Check sheet for the modelled part. Datum: model origin and axes. Units: mm. Face numbers are marked on the shaded views. A direction names the side the tool comes from. Round coordinates to 2 decimals unless told otherwise and drop trailing zeros. Order: outer loops, then holes, each group sorted by start corner. A loop starts at its lowest first (then second) coordinate and runs counter-clockwise, first axis right, second up.
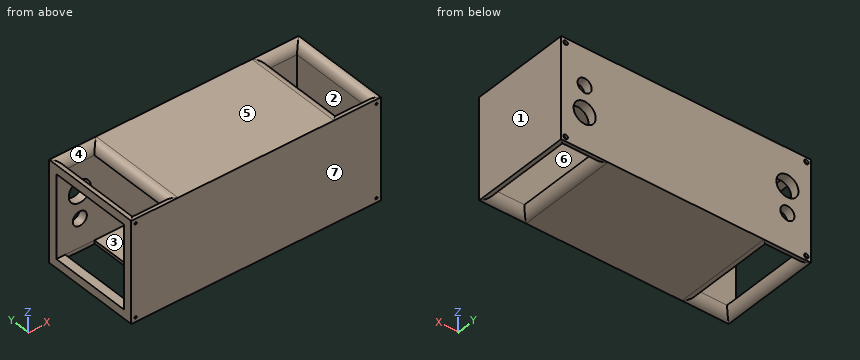
```python
from build123d import *

# Parameters (mm, degrees)
SKETCH1_W           = 282.5
SKETCH1_H           = 114
BOSS_EXTRUDE1_DEPTH = 114
SKETCH5_W           = 33
SKETCH5_H           = 94
CUT_EXTRUDE3_DEPTH  = 326.266429255
SKETCH6_W           = 94
SKETCH6_H           = 94
CUT_EXTRUDE4_DEPTH  = 262
SKETCH7_R           = 1.25
CUT_EXTRUDE5_DEPTH  = 262
SKETCH8_R           = 2.5
CUT_EXTRUDE6_DEPTH  = 2.5
FILLET3_R           = 10
FILLET4_R           = 10
FILLET6_R           = 10
SKETCH11_R          = 8
SKETCH11_R_2        = 12.5
CUT_EXTRUDE7_DEPTH  = 10


with BuildPart() as part:
    # Sketch1 → Boss-Extrude1 (new body)
    with BuildSketch(Plane.XY):
        with Locations((-141.25, 57)):
            Rectangle(SKETCH1_W, SKETCH1_H)
    extrude(amount=BOSS_EXTRUDE1_DEPTH)

    # Sketch5 → Cut-Extrude3 (cut, through all)
    with BuildSketch(Plane.XY):
        with Locations((-256, 57)):
            Rectangle(SKETCH5_W, SKETCH5_H)
        with Locations((-26.5, 57)):
            Rectangle(SKETCH5_W, SKETCH5_H)
    extrude(amount=CUT_EXTRUDE3_DEPTH, mode=Mode.SUBTRACT)

    # Sketch6 → Cut-Extrude4 (cut)
    with BuildSketch(Plane.ZY.offset(282.5)):
        with Locations((57, 57)):
            Rectangle(SKETCH6_W, SKETCH6_H)
    extrude(amount=-CUT_EXTRUDE4_DEPTH, mode=Mode.SUBTRACT)

    # Sketch7 → Cut-Extrude5 (cut)
    with BuildSketch(Plane(origin=(0, 114, 0), x_dir=(1, 0, 0), z_dir=(0, 1, 0))):
        with Locations(Location((-277.5, -109, 0), (0, 0, 180))):
            Circle(SKETCH7_R)
        with Locations(Location((-277.5, -5, 0), (0, 0, 180))):
            Circle(SKETCH7_R)
        with Locations(Location((-5, -109, 0), (0, 0, 180))):
            Circle(SKETCH7_R)
        with Locations(Location((-5, -5, 0), (0, 0, 180))):
            Circle(SKETCH7_R)
    extrude(amount=-CUT_EXTRUDE5_DEPTH, mode=Mode.SUBTRACT)

    # Sketch8 → Cut-Extrude6 (cut)
    with BuildSketch(Plane(origin=(0, 114, 0), x_dir=(1, 0, 0), z_dir=(0, 1, 0))):
        with Locations(Location((-277.5, -5, 0), (0, 0, 180))):
            Circle(SKETCH8_R)
        with Locations((-277.5, -109)):
            Circle(SKETCH8_R)
        with Locations((-5, -5)):
            Circle(SKETCH8_R)
        with Locations(Location((-5, -109, 0), (0, 0, 180))):
            Circle(SKETCH8_R)
    extrude(amount=-CUT_EXTRUDE6_DEPTH, mode=Mode.SUBTRACT)

    # Fillet3
    fillet3_edges = [part.edges().sort_by_distance(p)[0] for p in [
        (-256, 104, 114),
    ]]
    fillet(fillet3_edges, radius=FILLET3_R - 0.0001)  # a hair under: the kernel refuses the full size

    # Fillet4
    fillet4_edges = [part.edges().sort_by_distance(p)[0] for p in [
        (-239.5, 61.99995, 114),
        (-272.5, 61.99995, 114),
        (-256, 10, 114),
    ]]
    fillet(fillet4_edges, radius=FILLET4_R - 0.0001)  # a hair under: the kernel refuses the full size

    # Fillet6
    fillet6_edges = [part.edges().sort_by_distance(p)[0] for p in [
        (-256, 104, 0),
        (-239.5, 57, 0),
        (-272.5, 57, 0),
        (-256, 10, 0),
        (-26.5, 10, 0),
        (-10, 57, 0),
        (-43, 57, 0),
        (-26.5, 104, 0),
        (-26.5, 10, 114),
        (-26.5, 104, 114),
        (-10, 57, 114),
        (-43, 57, 114),
    ]]
    fillet(fillet6_edges, radius=FILLET6_R - 0.0001)  # a hair under: the kernel refuses the full size

    # Sketch11 → Cut-Extrude7 (cut)
    with BuildSketch(Plane(origin=(0, 114, 0), x_dir=(1, 0, 0), z_dir=(0, 1, 0))):
        with Locations(Location((-256, -42, 0), (0, 0, 180))):
            Circle(SKETCH11_R)
        with Locations(Location((-256, -72, 0), (0, 0, 180))):
            Circle(SKETCH11_R_2)
        with Locations(Location((-26.5, -42, 0), (0, 0, 180))):
            Circle(SKETCH11_R_2)
        with Locations(Location((-26.5, -72, 0), (0, 0, 180))):
            Circle(SKETCH11_R)
    extrude(amount=-CUT_EXTRUDE7_DEPTH, mode=Mode.SUBTRACT)


solid = part.part
```
Item 1: Sectioned sample at A-A (y = 60). State how many separate pieces and enclosed holes the cut face has, and give its area (3 significant figures).
Answer:
separate pieces: 5
enclosed holes: 4
area: 5,080 mm2
Item 2: Sectioned sample at D-D (z = 21). Record the cut outline in (x, y), and give its area (3 significant figures).
Answer:
outline: (-282.5, 0) - (0, 0) - (0, 114) - (-282.5, 114) - (-282.5, 104) - (-10, 104) - (-10, 10) - (-282.5, 10) - close
area: 6,590 mm2
Item 3: Release check for a two-part mould opening along Z. For the marked faces 5, 6 and 7 record: released by +Z, released by -Z, zero draft, split by the parting line, or undercut.
Answer:
face 5: released by +Z
face 6: undercut
face 7: zero draft
Item 4: Go/stop test with flat-tipped pins: P1, Ø6, axis at y = 54, z = 96.5, coming from the -X side; P2, Ø1.5, axis at y = 18.5, z = 63.5, coming from the +X side; P3, Ø22.5, axis at x = -26.5, z = 42, coming from the +Y side; P4, Ø4, axis at x = -277.5, z = 5, coming from the +Y side. Record where each tip stops, or that it passes through.
Answer:
P1: stops at x = -10
P2: stops at x = 0
P3: stops at y = 10
P4: stops at y = 111.5
Item 5: Access from +Z, -Z, +X, -X, +Y, -Y to the whole of each face (thin tool, end or side, straight path). Record for the marked faces 1, 2, 3 and 4.
Answer:
face 1: +Z, -Z, +X, +Y, -Y
face 2: +Z, -Z, -X
face 3: -X
face 4: +Z
Item 6: Sectioned sample at B-B (z = 42). Record the cut outline in (x, y).
Answer:
outline: (-282.5, 0) - (0, 0) - (0, 114) - (-14, 114) - (-14, 104) - (-10, 104) - (-10, 10) - (-282.5, 10) - close; (-282.5, 104) - (-264, 104) - (-264, 114) - (-282.5, 114) - close; (-248, 104) - (-39, 104) - (-39, 114) - (-248, 114) - close
Item 7: Scan lines: line 1 along Z through (x, y) = (-5, 112.95); line 2 along Y through (x, z) = (-69.5, 83); line 3 along Z through (x, y) = (-256, 106). Record each from-to range of solid material in increasing order.
Answer:
line 1: z = 0.06 to 2.5, 7.5 to 106.5, 111.5 to 113.94
line 2: y = 0 to 10, 104 to 114
line 3: z = 4 to 34, 50 to 59.5, 84.5 to 110
